Geometry check sheet. Reference: the model listing, model coordinates, mm. A direction names the side the tool comes from. Coordinates: 2 decimals unless noted, no trailing zeros. Write each loop counter-clockwise with the first axis right and the second up, starting at its lowest first coordinate (ties: lowest second). Pieces come first, ordered by that corner, then holes. Notation, with made-up numbers: (60, -31) -> (75, -31) arc R33 ccw to (75, -3) -> close; hole circle Ø3 at (19.25, 72.5). An arc over 180 degrees is marked (long way). Answer in a Markdown table with one row per item. Add a question column.
1. Set-up check for faces 1 (the flat face through (-30, -27.775, 5)), 2 (the flat face through (-2, 36, 0)): record each of +Z, -Z, +X, -X, +Y, -Y from which the full face is reachable in a straight line by a thin tool's end or side.
2. Cross-section at A-A on y = -24.5. Record the cut outline in (x, z), and give its area (4 significant figures).
3. Cross-section at C-C on y = 0. Record the cut outline in (x, z) (3 decimals).
4. Mould release check, pull along X, two halves, no side actions. Record for faces 3 (the flat face through (30, 0, 5)), 4 (the flat face through (-115, -1, 5)), 5 (the flat face through (-2, 36, 10)), 6 (the flat face through (-87.5, 0, 5)): pulls with the +X half, pulls with the -X half, needs draft (parallel to the pull), parting line crosses it, or undercut.
5. Cross-section at B-B on x = -9. Record the cut outline in (y, z) (3 decimals), and give its area (4 significant figures).
6. Depth check by flat-ended pin: P1, Ø11, axis at x = -96.225, y = 0, coming from the -Z side. Enter the tip coordinate at first touch or a pass-through.
7. Cross-section at D-D on z = 4.5. Record the cut outline in (x, y) (3 decimals), and give its area (3 significant figures).
8. Scan lines: L1, parallel to X at y = 2.5, z = 3.5; L2, parallel to X at y = -26, z = 8.5; L3, parallel to Y at x = 1, z = 1 (3 decimals). Record each from-to range of solid material in increasing order. Write a range as from..to.
```python
from build123d import *

# Parameters (mm, degrees)
SKETCH1_W           = 230
SKETCH1_H           = 105
BOSS_EXTRUDE1_DEPTH = 10
SKETCH2_R           = 6
SKETCH2_W           = 117.5
SKETCH2_H           = 55.55
CUT_EXTRUDE3_DEPTH  = 10


with BuildPart() as part:
    # Sketch1 → Boss-Extrude1 (new body)
    with BuildSketch(Plane.XY):
        Rectangle(SKETCH1_W, SKETCH1_H)
    extrude(amount=BOSS_EXTRUDE1_DEPTH)

    # Sketch2 → Cut-Extrude3 (cut)
    with BuildSketch(Plane.XY.offset(10)):
        with Locations((38.725, 0)):
            Circle(SKETCH2_R)
        with Locations((-96.225, 0)):
            Circle(SKETCH2_R)
        with Locations((-28.75, 0)):
            Rectangle(SKETCH2_W, SKETCH2_H)
    extrude(amount=-CUT_EXTRUDE3_DEPTH, mode=Mode.SUBTRACT)


solid = part.part
```
Results found:
| question | item | result |
|---|---|---|
| 1 | face 1 | +Z, -Z |
| 1 | face 2 | -Z, +X, -X, +Y, -Y |
| 2 | outline | (-115, 0) -> (-87.5, 0) -> (-87.5, 10) -> (-115, 10) -> close; (30, 0) -> (115, 0) -> (115, 10) -> (30, 10) -> close |
| 2 | area | 1,125 mm^2 |
| 3 | outline | (-115, 0) -> (-102.225, 0) -> (-102.225, 10) -> (-115, 10) -> close; (-90.225, 0) -> (-87.5, 0) -> (-87.5, 10) -> (-90.225, 10) -> close; (30, 0) -> (32.725, 0) -> (32.725, 10) -> (30, 10) -> close; (44.725, 0) -> (115, 0) -> (115, 10) -> (44.725, 10) -> close |
| 4 | face 3 | undercut |
| 4 | face 4 | pulls with the -X half |
| 4 | face 5 | needs draft |
| 4 | face 6 | undercut |
| 5 | outline | (-52.5, 0) -> (-27.775, 0) -> (-27.775, 10) -> (-52.5, 10) -> close; (27.775, 0) -> (52.5, 0) -> (52.5, 10) -> (27.775, 10) -> close |
| 5 | area | 494.5 mm^2 |
| 6 | P1 | passes through |
| 7 | outline | (-115, -52.5) -> (115, -52.5) -> (115, 52.5) -> (-115, 52.5) -> close; hole circle Ø12 at (-96.225, 0); hole (-87.5, -27.775) -> (30, -27.775) -> (30, 27.775) -> (-87.5, 27.775) -> close; hole circle Ø12 at (38.725, 0) |
| 7 | area | 17,400 mm^2 |
| 8 | L1 | x = -115..-101.68, -90.77..-87.5, 30..33.27, 44.18..115 |
| 8 | L2 | x = -115..-87.5, 30..115 |
| 8 | L3 | y = -52.5..-27.775, 27.775..52.5 |
